from build123d import *

# Parameters (mm, degrees)
SKETCH1_R           = 1
BOSS_EXTRUDE1_DEPTH = 30
SKETCH1_2_R         = 1
DOME2_FACE_RADIUS   = 1
DOME2_HEIGHT        = 1


with BuildPart() as part:
    # Sketch1 → Boss-Extrude1 (new body)
    with BuildSketch(Plane.XY):
        Circle(SKETCH1_R)
    extrude(amount=-BOSS_EXTRUDE1_DEPTH)

    # Sweep1: sweep along a path in Sketch3
    with BuildLine(Plane(origin=(0, 0, 0), x_dir=(1, 0, 0), z_dir=(0, 1, 0))) as sweep1_path:
        Line((0, 0), (0, -2))
        ThreePointArc((0, -2), (-0.300326829, -3.054092553), (-1.111111111, -3.791612833))
        ThreePointArc((-1.111111111, -3.791612833), (-0.29627421, -8.513511116), (1.606969024, -4.116017766))
    # Sketch1<2> → Sweep1 (sweep)
    with BuildSketch(Plane.XY):
        Circle(SKETCH1_2_R)
    sweep(path=sweep1_path.line)

    # Dome2: a dome of height H over a round flat face of radius A is a cap of a sphere of radius (A * A + H * H) / (2 * H)
    dome2_r = (DOME2_FACE_RADIUS * DOME2_FACE_RADIUS + DOME2_HEIGHT * DOME2_HEIGHT) / (2 * DOME2_HEIGHT)
    dome2_base = Plane((1.606969024, 0, 4.116017766), z_dir=(-0.766044443119, 0, -0.642787609687))
    with Locations(dome2_base.offset(DOME2_HEIGHT - dome2_r)):
        dome2_ball = Sphere(dome2_r, mode=Mode.PRIVATE)
    add(split(dome2_ball, bisect_by=dome2_base, keep=Keep.TOP, mode=Mode.PRIVATE))


solid = part.part
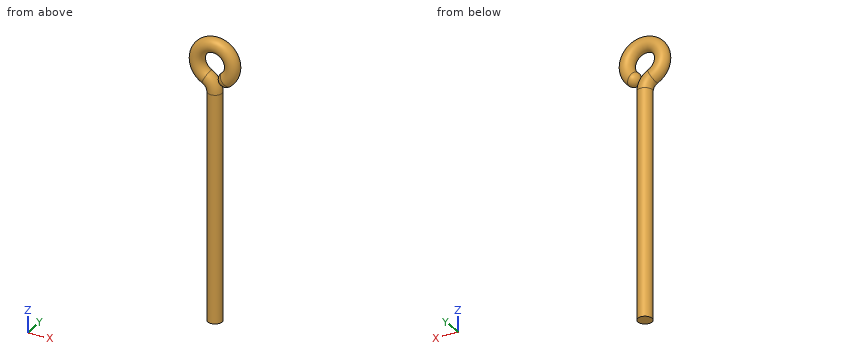
Input: part model. Units: mm. Frame: model coordinates. Round coordinates to 2 decimals unless told otherwise and drop trailing zeros. Order: outer loops, then holes, each group sorted by start corner. A loop starts at its lowest first (then second) coordinate and runs counter-clockwise, first axis right, second up.
1. Cut plane A-A, the plane y = 0. Output: boundary loops of the cut face in (x, z), then the cut area to 3 significant figures.
The answers:
outline: (-1.56, 2.9) arc R1 cw to (-1, 2) - (-1, -30) - (1, -30) - (1, 2) arc R3 ccw to (-0.67, 4.69) arc R1.5 cw (long way) to (0.96, 4.88) arc R1 ccw to (2.25, 3.35) arc R3.5 ccw (long way) to start
area: 95.6 mm2
2. Pin query (flat end, axial travel): P1, Ø1, axis at y = -0.5, z = -7.5, coming from the +X side. Return the tip coordinate at first contact, or that it passes through.
The answers:
P1: stops at x = 1
3. Cut plane B-B, the plane z = -3. Output: boundary loops of the cut face in (x, y).
The answers:
outline: circle Ø2 at (0, 0)
4. Material intervals for line 1 (X direction, y = 0.25, z = 4.5); line 2 (Z direction, x = 1.5, y = 0.8); line 3 (X direction, y = -0.1, z = -6), sorted ascending.
The answers:
line 1: x = -3.11 to -0.4, 0.72 to 3.11
line 2: z = 3.53 to 4.86, 7.2 to 8.74
line 3: x = -0.99 to 0.99
